from build123d import *

# Parameters (mm, degrees)
F0_W     = 13.46
F0_H     = 13.46
F0_R     = 5.742874
F1_DEPTH = 5.08
F0_W_2   = 17.6
F0_H_2   = 17.6
F2_DEPTH = 5.842
F3_DEPTH = 3.81


with BuildPart() as f1:
    # F0 (on Top) → F1 (new body)
    with BuildSketch(Plane.XY):
        Rectangle(F0_W, F0_H)
        Circle(F0_R, mode=Mode.SUBTRACT)
    extrude(amount=F1_DEPTH)

    # F0 (on Top) → F2 (join)
    with BuildSketch(Plane.XY):
        Rectangle(F0_W_2, F0_H_2)
        Rectangle(F0_W, F0_H, mode=Mode.SUBTRACT)
    extrude(amount=F2_DEPTH)

    # F0 (on Top) → F3 (join)
    with BuildSketch(Plane.XY):
        Circle(F0_R)
    extrude(amount=F3_DEPTH)


solid = f1.part
Could you check a few things on this model? Use its own coordinates, in mm. A direction names the side the tool comes from. Give positions to 0.01 mm unless a question says otherwise; leave off trailing zeros. Order: outer loops, then holes, each group sorted by start corner. A loop starts at its lowest first (then second) coordinate and runs counter-clockwise, first axis right, second up.
1. Suppose I cut it at A-A (x = -6). Write out the boundary of the cut face in (y, z).
Answers below:
outline: (-8.8, 0) - (8.8, 0) - (8.8, 5.84) - (6.73, 5.84) - (6.73, 5.08) - (-6.73, 5.08) - (-6.73, 5.84) - (-8.8, 5.84) - close
2. I need wall thicknesses on L1, parallel to Y at x = 0, z = 4.3; L2, parallel to X at y = 2.5, z = 5.25; L3, parallel to Z at x = 2.5, y = -2. Which ranges of each line are inside material? Lowest first, please.
Answers below:
L1: y = -8.8 to -5.74, 5.74 to 8.8
L2: x = -8.8 to -6.73, 6.73 to 8.8
L3: z = 0 to 3.81
3. For pin 1 (3.5 mm diameter, centred on x = 0, y = 0, fed in from +Z), with a flat end and sliding along its axis, tell me the tip position at first contact or that it passes through.
Answers below:
pin 1: stops at z = 3.81
4. Suppose I cut it at B-B (y = 0). Write out the boundary of the cut face in (x, z), plus the area to 3 significant figures.
Answers below:
outline: (-8.8, 0) - (8.8, 0) - (8.8, 5.84) - (6.73, 5.84) - (6.73, 5.08) - (5.74, 5.08) - (5.74, 3.81) - (-5.74, 3.81) - (-5.74, 5.08) - (-6.73, 5.08) - (-6.73, 5.84) - (-8.8, 5.84) - close
area: 78.0 mm2
5. Which directions (+Z, -Z, +X, -X, +Y, -Y) give clear straight access to the entire face, cutting with the end or side of a thin tool? Please do faces 4 (the flat face through (0, -8.8, 3)), 5 (the flat face through (6, 0, 5.08)).
Answers below:
face 4: +Z, -Z, +X, -X, -Y
face 5: +Z
6. Thinking about a two-plate mould opening in X: for faces 1 (the cylindrical face through (-1.245, -5.606, 4.436)), 2 (the flat face through (8.8, 0, 3)), 3 (the flat face through (0, 8.8, 3)), which applies, +X half, -X half, draft (parallel to the pull), parting line (faces both ways), or undercut?
Answers below:
face 1: undercut
face 2: +X half
face 3: draft
